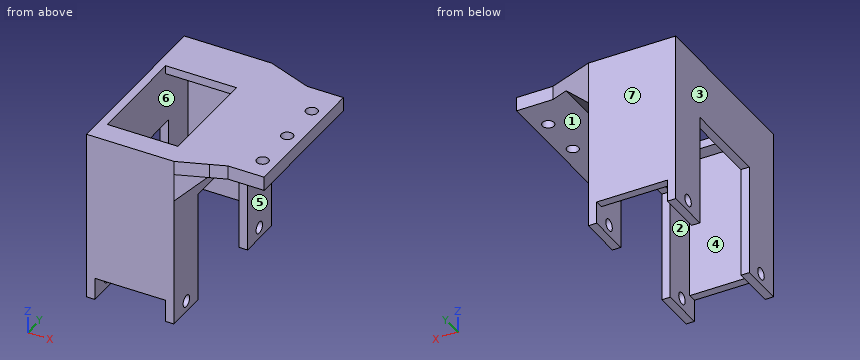
```python
from build123d import *

# Parameters (mm, degrees)
SKETCH1_W           = 51.2
SKETCH1_H           = 13
SKETCH1_R           = 2.1
SKETCH1_W_2         = 5
SKETCH1_H_2         = 25.4
BOSS_EXTRUDE1_DEPTH = 3
BOSS_EXTRUDE2_DEPTH = 61.6
SKETCH2_R           = 2.1
SKETCH2_W           = 32
SKETCH2_H           = 40
CUT_EXTRUDE1_DEPTH  = 100
SKETCH3_W           = 63.2
SKETCH3_H           = 25.4
CUT_EXTRUDE2_DEPTH  = 8
SKETCH1_5_W         = 51.2
SKETCH1_5_H         = 13
SKETCH1_5_R         = 2.1
BOSS_EXTRUDE3_DEPTH = 5
CHAMFER1_SIZE       = 10


with BuildPart() as part:
    # Sketch1 → Boss-Extrude1 (new body)
    # profile 1 of 9: a face of its own
    with BuildSketch(Plane(origin=(0, 0, 0), x_dir=(0, 1, 0), z_dir=(0, 0, 1))):
        with BuildLine():
            Line((41.3, -15.7), (27.654113618, -15.7))
            ThreePointArc((27.654113618, -15.7), (15.999687497, -27.481812167), (0, -31.8))
            Line((0, -31.8), (35.3, -31.8))
            Line((35.3, -31.8), (41.3, -15.7))
        make_face()
    # profile 2 of 9: a face of its own
    with BuildSketch(Plane(origin=(0, 0, 0), x_dir=(0, 1, 0), z_dir=(0, 0, 1))):
        with BuildLine():
            Line((27.654113618, -15.7), (-21.9, -15.7))
            Line((-21.9, -15.7), (-17.974836126, -26.232523063))
            ThreePointArc((-17.974836126, -26.232523063), (-9.408660016, -30.376259097), (0, -31.8))
            ThreePointArc((0, -31.8), (15.999687497, -27.481812167), (27.654113618, -15.7))
        make_face()
    # profile 3 of 9: a face of its own
    with BuildSketch(Plane(origin=(0, 0, 0), x_dir=(0, 1, 0), z_dir=(0, 0, 1))):
        with BuildLine():
            ThreePointArc((0, -31.8), (-9.408660016, -30.376259097), (-17.974836126, -26.232523063))
            Line((-17.974836126, -26.232523063), (-15.9, -31.8))
            Line((-15.9, -31.8), (0, -31.8))
        make_face()
    # profile 4 of 9: a face of its own
    with BuildSketch(Plane(origin=(0, 0, 0), x_dir=(0, 1, 0), z_dir=(0, 0, 1))):
        with Locations((9.7, -38.3)):
            Rectangle(SKETCH1_W, SKETCH1_H)
        with Locations(Location((23.85, -39.8, 0), (0, 0, 270))):
            Circle(SKETCH1_R, mode=Mode.SUBTRACT)
        with Locations(Location((7.95, -39.8, 0), (0, 0, 270))):
            Circle(SKETCH1_R, mode=Mode.SUBTRACT)
        with Locations(Location((-7.95, -39.8, 0), (0, 0, 270))):
            Circle(SKETCH1_R, mode=Mode.SUBTRACT)
    # profile 5 of 9: a face of its own
    with BuildSketch(Plane(origin=(0, 0, 0), x_dir=(0, 1, 0), z_dir=(0, 0, 1))):
        with BuildLine():
            ThreePointArc((29.153901969, -12.7), (28.443587304, -14.219786963), (27.654113618, -15.7))
            Line((27.654113618, -15.7), (41.3, -15.7))
            Line((41.3, -15.7), (41.3, 15.7))
            Line((41.3, 15.7), (27.654113618, 15.7))
            ThreePointArc((27.654113618, 15.7), (28.443587304, 14.219786963), (29.153901969, 12.7))
            Line((29.153901969, 12.7), (38.3, 12.7))
            Line((38.3, 12.7), (38.3, -12.7))
            Line((38.3, -12.7), (29.153901969, -12.7))
        make_face()
    # profile 6 of 9: a face of its own
    with BuildSketch(Plane(origin=(0, 0, 0), x_dir=(0, 1, 0), z_dir=(0, 0, 1))):
        with BuildLine():
            Line((-21.9, 15.7), (-21.9, -15.7))
            Line((-21.9, -15.7), (27.654113618, -15.7))
            ThreePointArc((27.654113618, -15.7), (28.443587304, -14.219786963), (29.153901969, -12.7))
            Line((29.153901969, -12.7), (23.85, -12.7))
            Line((23.85, -12.7), (-13.9, -12.7))
            Line((-13.9, -12.7), (-18.9, -12.7))
            Line((-18.9, -12.7), (-18.9, 12.7))
            Line((-18.9, 12.7), (-13.9, 12.7))
            Line((-13.9, 12.7), (23.85, 12.7))
            Line((23.85, 12.7), (29.153901969, 12.7))
            ThreePointArc((29.153901969, 12.7), (28.443587304, 14.219786963), (27.654113618, 15.7))
            Line((27.654113618, 15.7), (-21.9, 15.7))
        make_face()
    # profile 7 of 9: a face of its own
    with BuildSketch(Plane(origin=(0, 0, 0), x_dir=(0, 1, 0), z_dir=(0, 0, 1))):
        with BuildLine():
            Line((23.85, -12.7), (29.153901969, -12.7))
            ThreePointArc((29.153901969, -12.7), (31.131447787, -6.486367142), (31.8, 0))
            ThreePointArc((31.8, 0), (31.131447787, 6.486367142), (29.153901969, 12.7))
            Line((29.153901969, 12.7), (23.85, 12.7))
            Line((23.85, 12.7), (23.85, -12.7))
        make_face()
    # profile 8 of 9: a face of its own
    with BuildSketch(Plane(origin=(0, 0, 0), x_dir=(0, 1, 0), z_dir=(0, 0, 1))):
        with BuildLine():
            ThreePointArc((31.8, 0), (31.131447787, -6.486367142), (29.153901969, -12.7))
            Line((29.153901969, -12.7), (38.3, -12.7))
            Line((38.3, -12.7), (38.3, 12.7))
            Line((38.3, 12.7), (29.153901969, 12.7))
            ThreePointArc((29.153901969, 12.7), (31.131447787, 6.486367142), (31.8, 0))
        make_face()
    # profile 9 of 9: a face of its own
    with BuildSketch(Plane(origin=(0, 0, 0), x_dir=(0, 1, 0), z_dir=(0, 0, 1))):
        with Locations((-16.4, 0)):
            Rectangle(SKETCH1_W_2, SKETCH1_H_2)
    extrude(amount=-BOSS_EXTRUDE1_DEPTH)

    # Sketch1<4> → Boss-Extrude2 (add)
    with BuildSketch(Plane(origin=(0, 0, 0), x_dir=(0, 1, 0), z_dir=(0, 0, 1))):
        with BuildLine():
            ThreePointArc((29.153901969, -12.7), (28.443587304, -14.219786963), (27.654113618, -15.7))
            Line((27.654113618, -15.7), (41.3, -15.7))
            Line((41.3, -15.7), (41.3, 15.7))
            Line((41.3, 15.7), (27.654113618, 15.7))
            ThreePointArc((27.654113618, 15.7), (28.443587304, 14.219786963), (29.153901969, 12.7))
            Line((29.153901969, 12.7), (38.3, 12.7))
            Line((38.3, 12.7), (38.3, -12.7))
            Line((38.3, -12.7), (29.153901969, -12.7))
        make_face()
        with BuildLine():
            Line((-21.9, 15.7), (-21.9, -15.7))
            Line((-21.9, -15.7), (27.654113618, -15.7))
            ThreePointArc((27.654113618, -15.7), (28.443587304, -14.219786963), (29.153901969, -12.7))
            Line((29.153901969, -12.7), (23.85, -12.7))
            Line((23.85, -12.7), (-13.9, -12.7))
            Line((-13.9, -12.7), (-18.9, -12.7))
            Line((-18.9, -12.7), (-18.9, 12.7))
            Line((-18.9, 12.7), (-13.9, 12.7))
            Line((-13.9, 12.7), (23.85, 12.7))
            Line((23.85, 12.7), (29.153901969, 12.7))
            ThreePointArc((29.153901969, 12.7), (28.443587304, 14.219786963), (27.654113618, 15.7))
            Line((27.654113618, 15.7), (-21.9, 15.7))
        make_face()
    extrude(amount=-BOSS_EXTRUDE2_DEPTH)

    # Sketch2 → Cut-Extrude1 (cut)
    with BuildSketch(Plane(origin=(-15.7, 0, 0), x_dir=(0, -1, 0), z_dir=(-1, 0, 0))):
        with Locations(Location((13.9, -57.6, 0), (0, 0, 270))):
            Circle(SKETCH2_R)
        with Locations(Location((-33.3, -57.6, 0), (0, 0, 270))):
            Circle(SKETCH2_R)
        with Locations((-9.7, -41.6)):
            Rectangle(SKETCH2_W, SKETCH2_H)
    extrude(amount=-CUT_EXTRUDE1_DEPTH, mode=Mode.SUBTRACT)

    # Sketch3 → Cut-Extrude2 (cut)
    with BuildSketch(Plane.YX.offset(61.6)):
        with Locations((9.7, 0)):
            Rectangle(SKETCH3_W, SKETCH3_H)
    extrude(amount=-CUT_EXTRUDE2_DEPTH, mode=Mode.SUBTRACT)

    # Sketch1<5> → Boss-Extrude3 (add)
    # profile 1 of 4: a face of its own
    with BuildSketch(Plane(origin=(0, 0, 0), x_dir=(0, 1, 0), z_dir=(0, 0, 1))):
        with BuildLine():
            Line((27.654113618, -15.7), (-21.9, -15.7))
            Line((-21.9, -15.7), (-17.974836126, -26.232523063))
            ThreePointArc((-17.974836126, -26.232523063), (-9.408660016, -30.376259097), (0, -31.8))
            ThreePointArc((0, -31.8), (15.999687497, -27.481812167), (27.654113618, -15.7))
        make_face()
    # profile 2 of 4: a face of its own
    with BuildSketch(Plane(origin=(0, 0, 0), x_dir=(0, 1, 0), z_dir=(0, 0, 1))):
        with BuildLine():
            Line((41.3, -15.7), (27.654113618, -15.7))
            ThreePointArc((27.654113618, -15.7), (15.999687497, -27.481812167), (0, -31.8))
            Line((0, -31.8), (35.3, -31.8))
            Line((35.3, -31.8), (41.3, -15.7))
        make_face()
    # profile 3 of 4: a face of its own
    with BuildSketch(Plane(origin=(0, 0, 0), x_dir=(0, 1, 0), z_dir=(0, 0, 1))):
        with BuildLine():
            ThreePointArc((0, -31.8), (-9.408660016, -30.376259097), (-17.974836126, -26.232523063))
            Line((-17.974836126, -26.232523063), (-15.9, -31.8))
            Line((-15.9, -31.8), (0, -31.8))
        make_face()
    # profile 4 of 4: a face of its own
    with BuildSketch(Plane(origin=(0, 0, 0), x_dir=(0, 1, 0), z_dir=(0, 0, 1))):
        with Locations((9.7, -38.3)):
            Rectangle(SKETCH1_5_W, SKETCH1_5_H)
        with Locations(Location((23.85, -39.8, 0), (0, 0, 270))):
            Circle(SKETCH1_5_R, mode=Mode.SUBTRACT)
        with Locations(Location((7.95, -39.8, 0), (0, 0, 270))):
            Circle(SKETCH1_5_R, mode=Mode.SUBTRACT)
        with Locations(Location((-7.95, -39.8, 0), (0, 0, 270))):
            Circle(SKETCH1_5_R, mode=Mode.SUBTRACT)
    extrude(amount=-BOSS_EXTRUDE3_DEPTH)

    # Chamfer1
    # the kernel refuses this chamfer: 10 mm, written as the material it adds along each edge
    with BuildSketch(Plane(origin=(15.7, -21.9, -5), x_dir=(-0.027495876610586317, 0, -0.9996219169112968), z_dir=(0, 1, 0))) as chamfer1_piece_1_section:
        Polygon((CHAMFER1_SIZE * 0.999621916911, -CHAMFER1_SIZE * 0.0274958766106), (-CHAMFER1_SIZE * 0.0274958766106, -CHAMFER1_SIZE * 0.999621916911), (0, 0), align=None)
    chamfer1_piece_1 = extrude(amount=63.2, mode=Mode.PRIVATE)
    chamfer1_piece_1 = split(chamfer1_piece_1, bisect_by=Plane(origin=(28.867881951, -16.992714801, -8.339298449), z_dir=(-0.34920923314434543, 0.9370447756039934, 0)), keep=Keep.TOP, mode=Mode.PRIVATE)
    chamfer1_piece_1 = split(chamfer1_piece_1, bisect_by=Plane(origin=(28.867881951, 36.392714801, -8.339298449), z_dir=(-0.3492092331443461, -0.9370447756039931, 0)), keep=Keep.TOP, mode=Mode.PRIVATE)
    add(chamfer1_piece_1)


solid = part.part
```
Check sheet for the modelled part. Datum: model origin and axes. Units: mm. Face numbers are marked on the shaded views. A direction names the side the tool comes from. Coordinates: 2 decimals unless noted, no trailing zeros. Loops run counter-clockwise (first coordinate to the right, second up) from the corner with the lowest first, then second, coordinate; pieces in that order, holes last.
1) Release check for a two-part mould opening along X. For the marked faces 4, 5, 6 and 7 record: released by +X, released by -X, zero draft, split by the parting line, or undercut.
2) Access from +Z, -Z, +X, -X, +Y, -Y to the whole of each face (thin tool, end or side, straight path). Record for the marked faces 1, 2 and 3.
3) Material ranges on probe 1 along Y at (x, z) = (13.9, -57.6); probe 2 along Y at (x, z) = (10, -16); probe 3 along X at (y, z) = (24.5, -15.5), recorded low to high.
4) Sectioned sample at B-B (z = -57.6). Count the separate pieces of the cut face and the enclosed holes in it, and give its area (3 significant figures).
5) Sectioned sample at A-A (x = 3). Record the boundary of the cut face in (y, z), and give its area (3 significant figures).
6) Sectioned sample at C-C (y = -7.95). Record the boundary of the cut face in (x, z).
7) Gauge pin test, flat ends, axial feed: pin 1 (1.5 mm diameter, centred on y = 11.5, z = -16.5, fed in from +X); pin 2 (12 mm diameter, centred on x = 20, y = 21, fed in from -Z); pin 3 (1.5 mm diameter, centred on x = 0, y = 39.5, fed in from -Z); pin 4 (6.5 mm diameter, centred on x = 39.8, y = 7.95, fed in from +Z). Record the tip position at first contact, or that the pin passes through.
8) Sectioned sample at D-D (z = -51). Record the boundary of the cut face in (x, y), and give its area (3 significant figures).
Check sheet entries:
1. face 4: undercut
1. face 5: released by +X
1. face 6: undercut
1. face 7: zero draft
2. face 1: -Z, +X, +Y, -Y
2. face 2: -Z
2. face 3: +Z, -Z, -X, +Y, -Y
3. probe 1: y = -21.9 to -16, -11.8 to -6.3, 25.7 to 31.2, 35.4 to 41.3
3. probe 2: y = -21.9 to -18.9, 38.3 to 41.3
3. probe 3: x = -15.7 to -12.7, 12.7 to 15.7
4. separate pieces: 8
4. enclosed holes: 0
4. area: 137 mm2
5. outline: (-21.9, -53.6) - (-18.9, -53.6) - (-18.9, -3) - (-13.9, -3) - (-13.9, 0) - (-21.9, 0) - close; (23.85, -3) - (38.3, -3) - (38.3, -53.6) - (41.3, -53.6) - (41.3, 0) - (23.85, 0) - close
5. area: 380 mm2
6. outline: (-15.7, -61.6) - (-12.7, -61.6) - (-12.7, 0) - (-15.7, 0) - close; (12.7, -61.6) - (15.7, -61.6) - (15.7, -15) - (25.7, -5) - (37.7, -5) - (37.7, 0) - (12.7, 0) - close; (41.9, -5) - (44.8, -5) - (44.8, 0) - (41.9, 0) - close
7. pin 1: stops at x = 15.7
7. pin 2: stops at z = -21.6
7. pin 3: stops at z = -53.6
7. pin 4: stops at z = 0
8. outline: (-15.7, -21.9) - (15.7, -21.9) - (15.7, -6.3) - (12.7, -6.3) - (12.7, -18.9) - (-12.7, -18.9) - (-12.7, -6.3) - (-15.7, -6.3) - close; (-15.7, 25.7) - (-12.7, 25.7) - (-12.7, 38.3) - (12.7, 38.3) - (12.7, 25.7) - (15.7, 25.7) - (15.7, 41.3) - (-15.7, 41.3) - close
8. area: 340 mm2
